The model under review builds one solid part; all positions refer to its coordinate system, in mm. Round coordinates to 2 decimals unless told otherwise and drop trailing zeros. Write each loop counter-clockwise with the first axis right and the second up, starting at its lowest first coordinate (ties: lowest second). Pieces come first, ordered by that corner, then holes. Notation, with made-up numbers: M 38,13 L 84,13 A29 ccw 84,39 Z; hole C 84.25,57 d9. An arc over 180 degrees is marked long. One line per item, written item: value. Start each with the question number.
1) For P1, Ø6, axis at y = 3.5, z = 48, coming from the -X side, flat-tipped, find the tip position at first contact; note if it passes through.
2) Mouldability with a two-part tool opening along X and no side actions: class faces 1 (the face through (-1.301, -5.857, 59.16)), 2 (the face through (0.38, -0.08, 56.19)), 3 (the face through (0, 0, 120)) as +X half, -X half, draft (parallel to the pull), parting line (faces both ways), or undercut.
3) Take a section at A-A, the plane y = 0. Write out the cut boundary in (x, z), and give its area (3 significant figures).
4) Take a section at D-D, the plane y = -4.75. Write out the cut boundary in (x, z).
5) Take a section at B-B, the plane x = 0. Write out the cut boundary in (y, z), and give its area (3 significant figures).
6) Wall thickness on probe 1 along X at (y, z) = (-0.25, 65); probe 2 along X at (y, z) = (3.5, 65); probe 3 along X at (y, z) = (2.5, 57.5): over which ranges is each line inside the solid? List them lowest first.
7) Take a section at C-C, the plane z = 65. Write out the cut boundary in (x, y), and give its area (3 significant figures).
from build123d import *

# Parameters (mm, degrees)
SKETCH1_R               = 6
BOSS_EXTRUDE1_DEPTH     = 120
CUT_EXTRUDE2_DEPTH      = 121.299625935
CUT_EXTRUDE2_DEPTH_BACK = 121.299625935
SKETCH12_R              = 1.25


with BuildPart() as part:
    # Sketch1 → Boss-Extrude1 (new body)
    with BuildSketch(Plane.XY):
        Circle(SKETCH1_R)
    extrude(amount=BOSS_EXTRUDE1_DEPTH)

    # Sketch12 → Cut-Extrude2 (cut, two sides: drawn at the far end of the back side and taken through both)
    with BuildSketch(Plane(origin=(0, 0, 0), x_dir=(1, 0, 0), z_dir=(0, 1, 0)).offset(-CUT_EXTRUDE2_DEPTH_BACK)):
        with Locations(Location((0, -5, 0), (0, 0, 270))):
            Circle(SKETCH12_R)
        with Locations(Location((0, -10, 0), (0, 0, 270))):
            Circle(SKETCH12_R)
        with Locations(Location((0, -65, 0), (0, 0, 270))):
            Circle(SKETCH12_R)
        with Locations(Location((0, -55, 0), (0, 0, 270))):
            Circle(SKETCH12_R)
        with Locations(Location((0, -110, 0), (0, 0, 270))):
            Circle(SKETCH12_R)
        with Locations(Location((0, -115, 0), (0, 0, 270))):
            Circle(SKETCH12_R)
    extrude(amount=CUT_EXTRUDE2_DEPTH + CUT_EXTRUDE2_DEPTH_BACK, mode=Mode.SUBTRACT)


solid = part.part
Checked values:
1. P1: stops at x = -5.98
2. face 1: parting line
2. face 2: undercut
2. face 3: draft
3. outline: M -6,0 L 6,0 L 6,120 L -6,120 Z; hole C 0,5 d2.5; hole C 0,10 d2.5; hole C 0,55 d2.5; hole C 0,65 d2.5; hole C 0,110 d2.5; hole C 0,115 d2.5
3. area: 1,410 mm2
4. outline: M -3.67,0 L 3.67,0 L 3.67,120 L -3.67,120 Z; hole C 0,5 d2.5; hole C 0,10 d2.5; hole C 0,55 d2.5; hole C 0,65 d2.5; hole C 0,110 d2.5; hole C 0,115 d2.5
5. outline: M -6,0 L 6,0 L 6,3.75 L -6,3.75 Z; M -6,6.25 L 6,6.25 L 6,8.75 L -6,8.75 Z; M -6,11.25 L 6,11.25 L 6,53.75 L -6,53.75 Z; M -6,56.25 L 6,56.25 L 6,63.75 L -6,63.75 Z; M -6,66.25 L 6,66.25 L 6,108.75 L -6,108.75 Z; M -6,111.25 L 6,111.25 L 6,113.75 L -6,113.75 Z; M -6,116.25 L 6,116.25 L 6,120 L -6,120 Z
5. area: 1,260 mm2
6. probe 1: x = -5.99 to -1.25, 1.25 to 5.99
6. probe 2: x = -4.87 to -1.25, 1.25 to 4.87
6. probe 3: x = -5.45 to 5.45
7. outline: M -1.25,-5.87 L -1.25,5.87 A6 ccw Z; M 1.25,-5.87 A6 ccw 1.25,5.87 Z
7. area: 83.3 mm2
